Verification items for the finished model (mm, model axes). Face numbers are marked on the shaded views. A direction names the side the tool comes from. Coordinates: 2 decimals unless noted, no trailing zeros. Write each loop counter-clockwise with the first axis right and the second up, starting at its lowest first coordinate (ties: lowest second). Pieces come first, ordered by that corner, then holes.
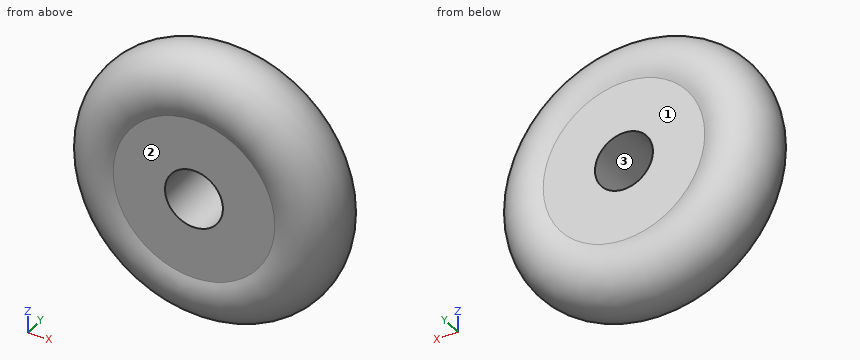
```python
from build123d import *

# Parameters (mm, degrees)
F0_R     = 7
F1_DEPTH = 5
F2_R     = 2.75
F4_R     = 2.1
F5_DEPTH = 5.251


with BuildPart() as f1:
    # F0 (on Front) → F1 (new body)
    with BuildSketch(Plane.XZ):
        Circle(F0_R)
    extrude(amount=F1_DEPTH)

    # F2 (on Top) → F3 (revolve)
    with BuildSketch(Plane.XY):
        with Locations((-7, -2.5)):
            Circle(F2_R)
    revolve(axis=Axis((0, -5, 0), (0, -1, 0)))

    # F4 (on face) → F5 (cut, through all)
    with BuildSketch(Plane.XZ.offset(5)):
        Circle(F4_R)
    extrude(amount=-F5_DEPTH, mode=Mode.SUBTRACT)


solid = f1.part
```
1. Sectioned sample at C-C, the plane y = -0.3. Record the boundary of the cut face in (x, z).
2. Gauge pin test, flat ends, axial feed: P1, Ø1.5, axis at y = -4.5, z = 6.5, coming from the +X side; P2, Ø4, axis at x = 0, z = -3.5, coming from the -Y side; P3, Ø2, axis at y = -1, z = -3, coming from the +X side; P4, Ø4, axis at x = 0, z = 0, coming from the -Y side. Record the tip position at first contact, or that the pin passes through.
3. Material ranges on L1, parallel to Y at x = -1.75, z = 3.5; L2, parallel to X at y = -3.65, z = 1; L3, parallel to Z at x = 1.75, y = -1.6, recorded low to high.
4. Sectioned sample at D-D, the plane y = -3.4. Record the boundary of the cut face in (x, z), and give its area (3 significant figures).
5. Tool access check on the marked faces 1, 2 and 3. Record the directions out of +Z, -Z, +X, -X, +Y, -Y that give a thin tool (end or side, any length) a straight path to the whole face; none if there is none.
6. Sectioned sample at A-A, the plane z = 0. Record the boundary of the cut face in (x, y).
7. Sectioned sample at B-B, the plane x = 0. Record the boundary of the cut face in (y, z).
Outcome:
1. outline: circle Ø17.3 at (0, 0); hole circle Ø4.2 at (0, 0)
2. P1: stops at x = 7.16
2. P2: stops at y = -5
2. P3: stops at x = 9.36
2. P4: passes through
3. L1: y = -5 to 0
3. L2: x = -9.45 to -1.85, 1.85 to 9.45
3. L3: z = -9.44 to -1.16, 1.16 to 9.44
4. outline: circle Ø19.2 at (0, 0); hole circle Ø4.2 at (0, 0)
4. area: 276 mm2
5. face 1: +Y
5. face 2: -Y
5. face 3: +Y, -Y
6. outline: (-5.85, -5) - (-2.1, -5) - (-2.1, 0) - (-5.85, 0) arc R2.75 ccw (long way) to start; (2.1, -5) - (5.85, -5) arc R2.75 ccw (long way) to (5.85, 0) - (2.1, 0) - close
7. outline: (-5, -5.85) arc R2.75 ccw (long way) to (0, -5.85) - (0, -2.1) - (-5, -2.1) - close; (-5, 2.1) - (0, 2.1) - (0, 5.85) arc R2.75 ccw (long way) to (-5, 5.85) - close
